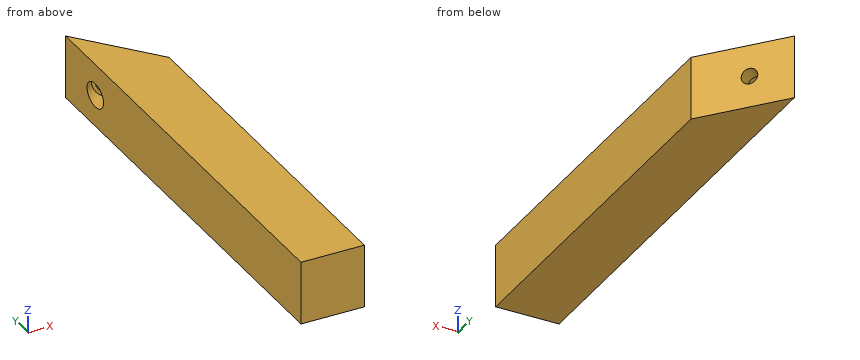
from build123d import *

# Parameters (mm, degrees)
F0_W     = 12.7
F0_H     = 12.7
F1_DEPTH = 177.8
F3_DEPTH = 25.401
F4_R     = 3.175
F5_DEPTH = 114.2886370023
F7_R     = 4.7625
F7_R_2   = 3.175
F8_DEPTH = 25.4


with BuildPart() as f1:
    # F0 (on Front) → F1 (new body)
    with BuildSketch(Plane.XZ):
        Polygon((12.7, -12.7), (12.7, 12.7), (-12.7, 12.7), (-12.7, -12.7), (-6.35, -12.7), (-6.35, 0), (6.35, 0), (6.35, -12.7), align=None)
        with Locations((0, -6.35)):
            Rectangle(F0_W, F0_H)
    extrude(amount=F1_DEPTH)

    # F2 (on face) → F3 (cut, through all)
    with BuildSketch(Plane.XY.offset(12.7)):
        Polygon((12.7, 0), (-12.7, 0), (12.7, -30.2705412519), align=None)
    extrude(amount=-F3_DEPTH, mode=Mode.SUBTRACT)

    # F4 (on face) → F5 (cut, through all)
    with BuildSketch(Plane(origin=(-7.4526659282, -6.2535292316, 0), x_dir=(-0.6427876097, 0.7660444431, 0), z_dir=(0.7660444431, 0.6427876097, 0))):
        with Locations((-8.981597357, 0)):
            Circle(F4_R)
    extrude(amount=-F5_DEPTH, mode=Mode.SUBTRACT)

    # F7 (on offset) → F8 (cut)
    with BuildSketch(Plane(origin=(-31.7745769972, -26.6620358392, 0), x_dir=(-0.6427876097, 0.7660444431, 0), z_dir=(0.7660444431, 0.6427876097, 0))):
        with Locations((-8.981597357, 0)):
            Circle(F7_R)
        with Locations((-8.981597357, 0)):
            Circle(F7_R_2, mode=Mode.SUBTRACT)
        with Locations((-8.981597357, 0)):
            Circle(F7_R_2)
    extrude(amount=F8_DEPTH, mode=Mode.SUBTRACT)


solid = f1.part
Can you work these out from the model? Positions are in its coordinate system, mm. Give positions to 0.01 mm unless a question says otherwise; leave off trailing zeros. Order: outer loops, then holes, each group sorted by start corner. A loop starts at its lowest first (then second) coordinate and runs counter-clockwise, first axis right, second up. Notation, with made-up numbers: M -34.75,-16.5 L 16.25,-16.5 A5 ccw 16.25,-9.5 Z; hole C 89.25,-36 d1. An arc over 180 degrees is marked long. Use a Markdown table: item, result. Add a question column.
Item 1: Will these pins go through, and if not, where does the flat tip stop? pin 1 (3 mm diameter, centred on x = -4, z = -4.5, fed in from +Y); pin 2 (10 mm diameter, centred on x = 5, z = -6, fed in from +Y); pin 3 (6 mm diameter, centred on x = 0.5, z = 1, fed in from +Y).
Item 2: Suppose I cut it at A-A (z = -9). List the corners of the cut face in (x, y) for me.
Item 3: Suppose I cut it at B-B (x = 7). List the corners of the cut face in (y, z) for me, then the cut area to 3 significant figures.
Item 4: If I drill on L1, parallel to Y at x = -7.75, z = -1.25; L2, parallel to Y at x = -10.5, z = 1; L3, parallel to Y at x = 3.5, z = 0, over which ranges is the centre line in solid material (lowest first)? Write a range as [from, to].
Answer sheet:
| question | item | result |
|---|---|---|
| 1 | pin 1 | stops at y = -8.58 |
| 1 | pin 2 | stops at y = -15.14 |
| 1 | pin 3 | stops at y = -13.26 |
| 2 | outline | M -12.7,-177.8 L 12.7,-177.8 L 12.7,-30.27 L -12.7,0 Z |
| 3 | outline | M -177.8,-12.7 L -23.48,-12.7 L -23.48,12.7 L -177.8,12.7 Z |
| 3 | area | 3,920 mm² |
| 4 | L1 | y = [-177.8, -24.23], [-14.42, -5.9] |
| 4 | L2 | y = [-177.8, -26.61], [-14.46, -2.62] |
| 4 | L3 | y = [-177.8, -19.31] |
